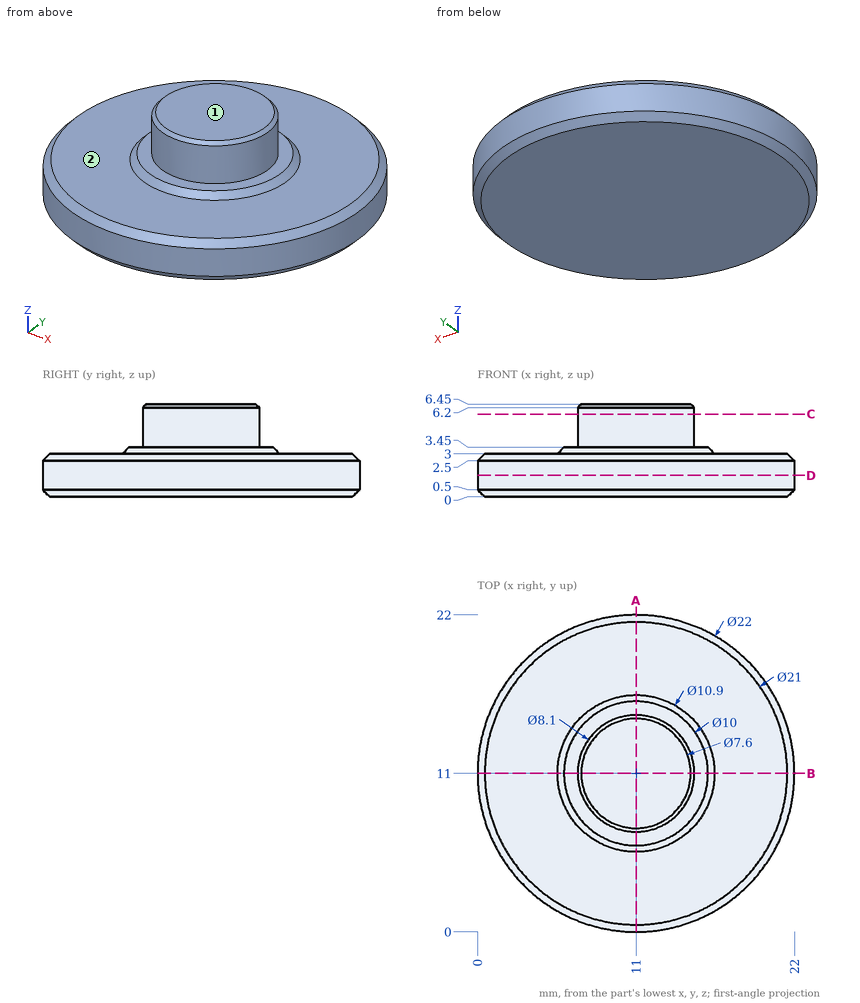
Source: three-view drawing plus pictorial views. Frame: mm from the lowest corner of the part. A direction names the side the tool comes from. Coordinates: 2 decimals unless noted, no trailing zeros. Write each loop counter-clockwise with the first axis right and the second up, starting at its lowest first coordinate (ties: lowest second). Pieces come first, ordered by that corner, then holes. Notation, with made-up numbers: (37.25, 13.25) -> (68.25, 13.25) arc R37 ccw to (68.25, 51.25) -> close; hole circle Ø4 at (-4.5, 49.25). An arc over 180 degrees is marked (long way). Write each question's results on one line, items separated by ' | '.
Item 1: Section query D-D on z = 1.5. Return loops of the section in (x, y), plus the area to 3 significant figures.
Conclusion:
outline: circle Ø22 at (11, 11) | area: 380 mm^2
Item 2: Section query A-A on x = 11. Return loops of the section in (y, z), plus the area to 3 significant figures.
Conclusion:
outline: (0, 0.5) -> (0.5, 0) -> (21.5, 0) -> (22, 0.5) -> (22, 2.5) -> (21.5, 3) -> (16.45, 3) -> (16, 3.45) -> (15.05, 3.45) -> (15.05, 6.2) -> (14.8, 6.45) -> (7.2, 6.45) -> (6.95, 6.2) -> (6.95, 3.45) -> (6, 3.45) -> (5.55, 3) -> (0.5, 3) -> (0, 2.5) -> close | area: 94.4 mm^2
Item 3: Pin query (flat end, axial travel): pin 1 Ø1 at (x, y) = (10.5, 17.5) entering from +Z; pin 2 Ø8 at (x, y) = (3, 11.5) entering from +Z. Return the tip coordinate at first contact, or that it passes through.
Conclusion:
pin 1: stops at z = 3 | pin 2: stops at z = 6.23
Item 4: Material intervals for probe 1 along Z at (x, y) = (2.5, 11.75); probe 2 along Z at (x, y) = (6.5, 11.75); probe 3 along X at (y, z) = (13.75, 1), sorted ascending.
Conclusion:
probe 1: z = 0 to 3 | probe 2: z = 0 to 3.45 | probe 3: x = 0.35 to 21.65
Item 5: Set-up query: the marked faces 1 and 2. Return all of +Z, -Z, +X, -X, +Y, -Y with unobstructed straight access to the full face (end or side cutting, diameter ignored); none if empty.
Conclusion:
face 1: +Z, +X, -X, +Y, -Y | face 2: +Z
Item 6: Section query C-C on z = 5.75. Return loops of the section in (x, y), plus the area to 3 significant figures.
Conclusion:
outline: circle Ø8.1 at (11, 11) | area: 51.5 mm^2
